The listing builds one solid part. Answer for the finished solid, in the listing's coordinates (mm). A direction names the side the tool comes from. Give positions to 0.01 mm unless a question says otherwise; leave off trailing zeros. Order: outer loops, then holes, each group sorted by start corner. A loop starts at its lowest first (then second) coordinate and runs counter-clockwise, first axis right, second up.
Autodesk Inventor part; units mm, degrees
ref_plane "YZ Plane" through (0, 0, 0) normal (1, 0, 0) x (0, 1, 0)
ref_plane "XZ Plane" through (0, 0, 0) normal (0, 1, 0) x (-1, 0, 0)
ref_plane "XY Plane" through (0, 0, 0) normal (0, 0, 1) x (1, 0, 0)
sketch "Boceto2" plane through (0, 0, 0) normal (0, 1, 0) x (-1, 0, 0)
  line L0 (0, 0) -> (243, 0)
  line L1 (243, 0) -> (243, -290)
  line L2 (243, -290) -> (0, -290)
  line L3 (0, -290) -> (0, 0)
  dimension "d4" = 243
  dimension "d5" = 290
extrude "Extrusión2" add sketch "Boceto2" along normal blind 61
sketch "Boceto3" plane through (0, 61, 0) normal (0, 1, 0) x (1, 0, 0)
  line L0 (0, 290) -> (-243, 290)
  line L1 (-243, 290) -> (-243, 0)
  line L2 (-243, 0) -> (0, 0)
  line L3 (0, 0) -> (0, 290)
  line L4 (-207, 36) -> (-207, 254)
  line L5 (-207, 254) -> (-36, 254)
  line L6 (-36, 254) -> (-36, 36)
  line L7 (-36, 36) -> (-207, 36)
  dimension "d8" = 36
sketch "Boceto4" plane through (0, 0, 0) normal (1, 0, 0) x (0, 0, -1)
  line L0 (0, 0) -> (290, 0)
  line L1 (290, 0) -> (290, 61)
  line L2 (0, 61) -> (290, 61)
  line L3 (0, 0) -> (0, 61)
  circle A0 centre (145, 30.5) radius 14.78
  dimension "d9" = 29.56
extrude "Extrusión3" cut sketch "Boceto4" against normal blind 69.75 contours A0
extrude "Extrusión4" cut sketch "Boceto3" against normal blind 46.25 contours L4 L5 L6 L7
properties part number "MADERA"
1) For a pull along X with two mould halves and no side action, classify faces 4 (the flat face through (-120, 0, -143)), 5 (the flat face through (-36, 48, -147)), 6 (the flat face through (0, 10, -147)), 7 (the flat face through (-123, 14.75, -147)) as +X half, -X half, draft (parallel to the pull), parting line (faces both ways), or undercut.
Geometry says:
face 4: draft
face 5: undercut
face 6: +X half
face 7: undercut
2) Find section C-C (x = -126). Write down the section's boundary in (y, z).
Geometry says:
outline: (0, -290) - (61, -290) - (61, -254) - (14.75, -254) - (14.75, -36) - (61, -36) - (61, 0) - (0, 0) - close
3) Find section A-A (z = -145). Write down the section's boundary in (x, y).
Geometry says:
outline: (-243, 0) - (0, 0) - (0, 15.72) - (-36, 15.72) - (-36, 14.75) - (-207, 14.75) - (-207, 61) - (-243, 61) - close; (-36, 45.28) - (0, 45.28) - (0, 61) - (-36, 61) - close
4) Find section D-D (z = -240). Write down the section's boundary in (x, y), then the cut area to 3 significant figures.
Geometry says:
outline: (-243, 0) - (0, 0) - (0, 61) - (-36, 61) - (-36, 14.75) - (-207, 14.75) - (-207, 61) - (-243, 61) - close
area: 6,910 mm2
5) Given P1, Ø1, axis at x = -140, z = -133, coming from the +Y side, flat-ended and moving along its own axis, determine where the tip first touches the part or whether it passes through.
Geometry says:
P1: stops at y = 14.75
6) Straight lines are drawn through the part: probe 1 along Y at (x, z) = (-23, -145); probe 2 along Z at (x, y) = (-109, 43.5); probe 3 along X at (y, z) = (41, -246). For each, find the intervals that lie inside material, in ascending order.
Geometry says:
probe 1: y = 0 to 15.72, 45.28 to 61
probe 2: z = -290 to -254, -36 to 0
probe 3: x = -243 to -207, -36 to 0
7) A tool of negligible diameter and unlimited length cuts with its end or side. For faces 1 (the flat face through (-12, 61, -143)), 2 (the cylindrical face through (-17.748, 31.15, -130.234)), 3 (the flat face through (-207, 38, -143)), from which of +Z, -Z, +X, -X, +Y, -Y can it reach the whole face along a straight path? Write none if from no direction.
Geometry says:
face 1: +Z, -Z, +X, -X, +Y
face 2: +X
face 3: +Y
8) Find section B-B (y = 30.5). Write down the section's boundary in (x, z), then the cut area to 3 significant figures.
Geometry says:
outline: (-243, -290) - (0, -290) - (0, -159.78) - (-36, -159.78) - (-36, -254) - (-207, -254) - (-207, -36) - (-36, -36) - (-36, -130.22) - (0, -130.22) - (0, 0) - (-243, 0) - close
area: 32,100 mm2
